Work out the finished part from the listing and answer in its coordinate system (mm). A direction names the side the tool comes from. Round coordinates to 2 decimals unless told otherwise and drop trailing zeros. Loops run counter-clockwise (first coordinate to the right, second up) from the corner with the lowest first, then second, coordinate; pieces in that order, holes last.
```python
from build123d import *

# Parameters (mm, degrees)
SKETCH1_W              = 44
SKETCH1_H              = 300
BASE_FLANGE1_DEPTH     = 1.2
SKETCHED_START         = -22
SKETCHED_BEND1_DEPTH   = 44
SKETCHED_BEND1_2_DEPTH = 44
SKETCH7_R              = 4
CUT_EXTRUDE1_DEPTH     = 10
SKETCH9_R              = 4.5
CUT_EXTRUDE2_DEPTH     = 10


# Read off the part's stored shape, not the designer's step: Sketched Bend1
# Sheet-metal steps are written as plain solids
with BuildPart() as part:
    # Sketch1 → Base-Flange1 (new body)
    with BuildSketch(Plane(origin=(0, 0, 0), x_dir=(1, 0, 0), z_dir=(0, 1, 0))):
        Rectangle(SKETCH1_W, SKETCH1_H)
    extrude(amount=-BASE_FLANGE1_DEPTH)

    # Sketched Bend1 outline → Sketched Bend1 (cut)
    with BuildSketch(Plane.YZ.offset(SKETCHED_START)):
        with BuildLine():
            ThreePointArc((-1.2, -110.7366), (-0.872269031, -109.658657516), (0, -108.945555612))
            Line((0, -108.945555612), (0, 150))
            Line((0, 150), (-1.2, 150))
            Line((-1.2, 150), (-1.2, -110.7366))
        make_face()
    extrude(amount=SKETCHED_BEND1_DEPTH, mode=Mode.SUBTRACT)

    # Sketched Bend1 2 outline → Sketched Bend1 2 (add)
    with BuildSketch(Plane.YZ.offset(SKETCHED_START)):
        with BuildLine():
            Line((257.6, -110), (257.6, -108.8))
            Line((257.6, -108.8), (0.7366, -108.8))
            ThreePointArc((0.7366, -108.8), (0.361178238, -108.836737358), (0, -108.945555612))
            Line((0, -108.945555612), (0, -110.7366))
            ThreePointArc((0, -110.7366), (0.215745145, -110.215745145), (0.7366, -110))
            Line((0.7366, -110), (257.6, -110))
        make_face()
    extrude(amount=SKETCHED_BEND1_2_DEPTH)

    # Sketch7 → Cut-Extrude1 (cut)
    with BuildSketch(Plane.XY.offset(-108.8)):
        with Locations((0, 72.8)):
            Circle(SKETCH7_R)
        with Locations((0, 212.8)):
            Circle(SKETCH7_R)
    extrude(amount=-CUT_EXTRUDE1_DEPTH, mode=Mode.SUBTRACT)

    # Sketch9 → Cut-Extrude2 (cut)
    with BuildSketch(Plane.XZ.offset(1.2)):
        with Locations(Location((0, -130.3683, 0), (0, 0, 270))):
            Circle(SKETCH9_R)
    extrude(amount=-CUT_EXTRUDE2_DEPTH, mode=Mode.SUBTRACT)


solid = part.part
```
1. Determine the mould class of faces 3 (the face through (-1.724, -0.608, -134.525)), 4 (the face through (22, 128, -109)), 5 (the face through (-0.31, 0, -135.01)), 6 (the face through (2.15, 216.173, -109.392)) for opening direction X: +X half, -X half, draft (parallel to the pull), parting line (faces both ways), or undercut.
Answer key:
face 3: undercut
face 4: +X half
face 5: draft
face 6: undercut
2. Find section C-C (z = -130). Write down the section's boundary in (x, y), then the cut area to 3 significant figures.
Answer key:
outline: (-22, -1.2) - (-4.48, -1.2) - (-4.48, 0) - (-22, 0) - close; (4.48, -1.2) - (22, -1.2) - (22, 0) - (4.48, 0) - close
area: 42.0 mm2
3. Which of the six approach directions +Z, -Z, +X, -X, +Y, -Y give full straight-line access (tool end or side, diameter ignored) to faces 1 (the face through (0, 127, -110)), 2 (the face through (-0.31, -1.2, -135.01))?
Answer key:
face 1: -Z, +X, -X, +Y
face 2: +Z, -Z, +X, -X, -Y
4. Find section D-D (x = 15). Write down the section's boundary in (y, z).
Answer key:
outline: (-1.2, -150) - (0, -150) - (0, -110.74) arc R0.74 cw to (0.74, -110) - (257.6, -110) - (257.6, -108.8) - (0.74, -108.8) arc R1.94 ccw to (-1.2, -110.74) - close
5. Consider probe 1 along Y at (x, z) = (0, -109); probe 2 along Y at (x, z) = (0, -109.3); probe 3 along Z at (x, y) = (-2, 29). Determine where each line is inside the solid, lowest interval first.
Answer key:
probe 1: y = -0.12 to 68.8, 76.8 to 208.8, 216.8 to 257.6
probe 2: y = -0.56 to 68.8, 76.8 to 208.8, 216.8 to 257.6
probe 3: z = -110 to -108.8
6. Given pin 1 (2 mm diameter, centred on x = 6.5, y = 73, fed in from -Z); pin 2 (3 mm diameter, centred on x = 1.5, y = 211.5, fed in from +Z), each flat-ended and moving along its own axis, determine where each tip first touches the part or whether it passes through.
Answer key:
pin 1: stops at z = -110
pin 2: passes through
7. Find section B-B (x = 0). Write down the section's boundary in (y, z).
Answer key:
outline: (-1.2, -150) - (0, -150) - (0, -134.87) - (-1.2, -134.87) - close; (-1.2, -125.87) - (0, -125.87) - (0, -110.74) arc R0.74 cw to (0.74, -110) - (68.8, -110) - (68.8, -108.8) - (0.74, -108.8) arc R1.94 ccw to (-1.2, -110.74) - close; (76.8, -110) - (208.8, -110) - (208.8, -108.8) - (76.8, -108.8) - close; (216.8, -110) - (257.6, -110) - (257.6, -108.8) - (216.8, -108.8) - close
8. Find section A-A (y = 212.8). Write down the section's boundary in (x, z), then the cut area to 3 significant figures.
Answer key:
outline: (-22, -110) - (-4, -110) - (-4, -108.8) - (-22, -108.8) - close; (4, -110) - (22, -110) - (22, -108.8) - (4, -108.8) - close
area: 43.2 mm2
